Here's how the part is built. I have some questions about the finished solid (model axes, mm). A direction names the side the tool comes from. Coordinates: 2 decimals unless noted, no trailing zeros. Order: outer loops, then holes, each group sorted by start corner. A loop starts at its lowest first (then second) coordinate and runs counter-clockwise, first axis right, second up. Notation, with made-up numbers: (32, 74) - (82, 74) arc R18 cw to (82, 100) - close; hole circle Ø6 at (61, 13.25). An arc over 180 degrees is marked (long way). Answer in a Markdown table with one row per item. Add a question column.
Item 1: On a 3-axis mill with a long thin cutter (end or side, diameter ignored), from which of +Z, -Z, +X, -X, +Y, -Y can I reach the whole of each face in a straight line? I mean faces 4 (the flat face through (4, -10, 6)), 5 (the flat face through (-17, -11, 6)), 6 (the flat face through (-28, -10, 6)). Say none if no direction works.
Item 2: I want a section at B-B (z = 8.75). Please give me the cut outline in (x, y), plus the area to 3 significant figures.
Item 3: I want a section at A-A (z = 2.75). Please give me the cut outline in (x, y), plus the area to 3 significant figures.
Item 4: I want a section at D-D (x = -27). Please give me the cut outline in (y, z), plus the area to 3 significant figures.
Item 5: Thinking about a two-plate mould opening in Y: for faces 1 (the flat face through (-18.3, -9.1, 2)), 2 (the cylindrical face through (17.48, -29.41, 6.04)), 3 (the flat face through (-41, -27, 10)), which applies, +Y half, -Y half, draft (parallel to the pull), parting line (faces both ways), or undercut?
Item 6: If I drill on line 1 along Z through (x, y) = (-26, -18); line 2 along Y through (x, z) = (11.5, 5.75); line 3 along X through (y, z) = (-7, 4), over which ranges is the centre line in solid material (lowest first)? Write a range as from..to.
Item 7: Will these pins go through, and if not, where does the flat tip stop? pin 1 Ø1 at (x, z) = (-9.5, 8) entering from +Y; pin 2 Ø4 at (y, z) = (-14.5, 2) entering from -X; pin 3 Ø6 at (x, z) = (-11, 4) entering from -Y.
Item 8: I want a section at C-C (y = 1). Please give me the cut outline in (x, z), plus the area to 3 significant figures.
```python
from build123d import *

# Parameters (mm, degrees)
SKETCH_1_R          = 5
SKETCH_1_R_2        = 2.5
EXTRUDE_1_DEPTH     = 10
EXTRUDE_1_2_DEPTH   = 10
EXTRUDE_1_3_DEPTH   = 10
EXTRUDE_2_DEPTH     = 6
EXTRUDE_4_DEPTH     = 6
CUT_EXTRUDE_1_DEPTH = 4
SKETCH_5_R          = 3.75
SKETCH_5_R_2        = 2.5
EXTRUDE_3_DEPTH     = 2
CUT_EXTRUDE_2_DEPTH = 4
CUT_EXTRUDE_3_DEPTH = 8
SKETCH_11_R         = 2.5
EXTRUDE_9_DEPTH     = 2


with BuildPart() as part:
    # Sketch 1 → Extrude 1 (new body)
    with BuildSketch(Plane.XY):
        with Locations((-12.085916667, 0.414052586)):
            Circle(SKETCH_1_R)
        with Locations((-12.085916667, 0.414052586)):
            Circle(SKETCH_1_R_2, mode=Mode.SUBTRACT)
    extrude(amount=EXTRUDE_1_DEPTH)



with BuildPart() as body_2:
    # Sketch 1 → Extrude 1 2 (new body)
    with BuildSketch(Plane.XY):
        with Locations((-38.24886757, -25.748898318)):
            Circle(SKETCH_1_R)
        with Locations((-38.24886757, -25.748898318)):
            Circle(SKETCH_1_R_2, mode=Mode.SUBTRACT)
    extrude(amount=EXTRUDE_1_2_DEPTH)


with BuildPart() as body_3:
    # Sketch 1 → Extrude 1 3 (new body)
    with BuildSketch(Plane.XY):
        with Locations((14.077034237, -25.748898318)):
            Circle(SKETCH_1_R)
        with Locations((14.077034237, -25.748898318)):
            Circle(SKETCH_1_R_2, mode=Mode.SUBTRACT)
    extrude(amount=EXTRUDE_1_3_DEPTH)


with BuildPart() as part_1:
    add(part.part)

    add(body_2.part)  # Extrude 2 merges body 2
    # Sketch 3 → Extrude 2 (add)
    with BuildSketch(Plane(origin=(0, 0, 0), x_dir=(-1, 0, 0), z_dir=(0, 0, -1))):
        Polygon((12.085916667, 0.414052586), (15.621450572, 3.949586492), (41.784401476, -22.213364412), (34.713333665, -29.284432224), (8.550382761, -3.12148132), align=None)
    extrude(amount=-EXTRUDE_2_DEPTH)


    add(body_3.part)  # Extrude 4 merges body 3
    # Sketch 9 → Extrude 4 (add)
    with BuildSketch(Plane(origin=(0, 0, 0), x_dir=(-1, 0, 0), z_dir=(0, 0, -1))):
        Polygon((-14.077034237, -25.748898318), (-17.612568143, -22.213364412), (8.550382761, 3.949586492), (15.621450572, -3.12148132), (-10.541500331, -29.284432224), align=None)
    extrude(amount=-EXTRUDE_4_DEPTH)

    # Sketch 4 → Cut-Extrude 1 (cut)
    with BuildSketch(Plane.XY.offset(6)):
        Polygon((-13.85368362, 2.181819539), (-10.318149714, -1.353714367), (-36.481100617, -27.516665271), (-40.016634523, -23.981131365), align=None)
    extrude(amount=-CUT_EXTRUDE_1_DEPTH, mode=Mode.SUBTRACT)

    # Sketch 5 → Extrude 3 (add)
    with BuildSketch(Plane(origin=(0, 0, 0), x_dir=(-1, 0, 0), z_dir=(0, 0, -1))):
        with Locations((12.969800143, 1.297936063)):
            Circle(SKETCH_5_R)
        with Locations(Location((38.24886757, -25.748898318, 0), (0, 0, 45))):
            Circle(SKETCH_5_R_2)
    extrude(amount=-EXTRUDE_3_DEPTH)

    # Sketch 4_2 → Cut-Extrude 2 (cut)
    with BuildSketch(Plane.XY.offset(6)):
        Polygon((-13.85368362, 2.181819539), (-10.318149714, -1.353714367), (-36.481100617, -27.516665271), (-40.016634523, -23.981131365), align=None)
    extrude(amount=CUT_EXTRUDE_2_DEPTH, mode=Mode.SUBTRACT)

    # Sketch 10 → Cut-Extrude 3 (cut)
    with BuildSketch(Plane.XY.offset(10)):
        Polygon((14.077034237, -25.748898318), (12.309267284, -27.516665271), (-13.85368362, -1.353714367), (-12.085916667, 0.414052586), (-10.318149714, 2.181819539), (15.84480119, -23.981131365), align=None)
    extrude(amount=-CUT_EXTRUDE_3_DEPTH, mode=Mode.SUBTRACT)

    # Sketch 11 → Extrude 9 (add)
    with BuildSketch(Plane(origin=(0, 0, 0), x_dir=(-1, 0, 0), z_dir=(0, 0, -1))):
        with Locations((-14.077034237, -25.748898318)):
            Circle(SKETCH_11_R)
    extrude(amount=-EXTRUDE_9_DEPTH)


solid = part_1.part
```
Values follow:
| question | item | result |
|---|---|---|
| 1 | face 4 | +Z, +X, +Y |
| 1 | face 5 | +Z, -Y |
| 1 | face 6 | +Z, -X, +Y |
| 2 | outline | (-40.02, -23.98) - (-36.95, -20.92) arc R5 ccw (long way) to (-33.42, -24.45) - (-36.48, -27.52) arc R2.5 cw to start; (-16.92, -0.88) - (-13.85, 2.18) arc R2.5 cw to (-10.32, 2.18) - (-7.26, -0.88) arc R5 ccw (long way) to start; (-13.38, -4.42) arc R5 ccw to (-10.79, -4.42) - (-12.09, -3.12) - close; (9.25, -24.45) arc R5 ccw (long way) to (12.78, -20.92) - (15.84, -23.98) arc R2.5 cw to (12.31, -27.52) - close |
| 2 | area | 122 mm^2 |
| 3 | outline | (-41.78, -22.21) arc R5 ccw to (-34.71, -29.28) - (-12.09, -6.66) - (10.54, -29.28) arc R5 ccw to (17.61, -22.21) - (-8.55, 3.95) arc R5 ccw to (-15.62, 3.95) - close; hole (-40.02, -23.98) arc R2.5 ccw to (-36.48, -27.52) - (-12.09, -3.12) - (12.31, -27.52) arc R2.5 ccw to (15.84, -23.98) - (-10.32, 2.18) arc R2.5 ccw to (-13.85, 2.18) - close |
| 3 | area | 425 mm^2 |
| 4 | outline | (-21.57, 0) - (-7.43, 0) - (-7.43, 6) - (-10.96, 6) - (-10.96, 2) - (-18.04, 2) - (-18.04, 6) - (-21.57, 6) - close |
| 4 | area | 56.6 mm^2 |
| 5 | face 1 | undercut |
| 5 | face 2 | parting line |
| 5 | face 3 | draft |
| 6 | line 1 | z = 0..6 |
| 6 | line 2 | y = -30.03..-26.71, -19.64..-16.1 |
| 6 | line 3 | x = -26.57..-23.04, -15.96..-12.43, -11.74..-8.21, -1.14..2.4 |
| 7 | pin 1 | stops at y = 4.96 |
| 7 | pin 2 | stops at x = -36.07 |
| 7 | pin 3 | stops at y = -10.74 |
| 8 | outline | (-18.57, 0) - (-5.6, 0) - (-5.6, 6) - (-7.12, 6) - (-7.12, 10) - (-9.14, 10) - (-9.14, 2) - (-15.04, 2) - (-15.04, 10) - (-17.05, 10) - (-17.05, 6) - (-18.57, 6) - close |
| 8 | area | 70.4 mm^2 |
